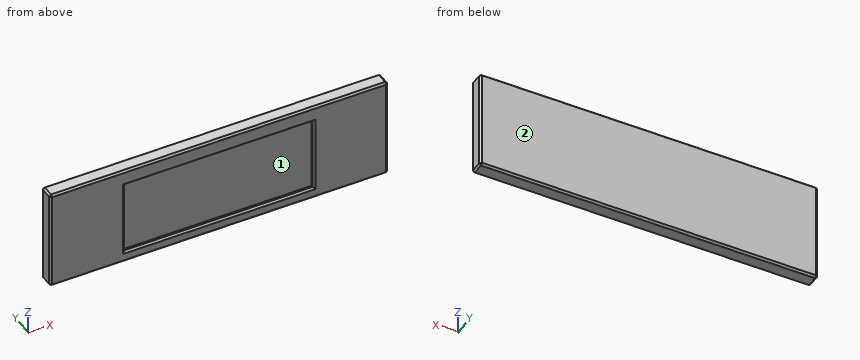
from build123d import *

# Parameters (mm, degrees)
F0_W     = 900
F0_H     = 270
F0_W_2   = 502
F0_H_2   = 197
F1_DEPTH = 40
F2_DEPTH = 30
F3_SIZE  = 5


with BuildPart() as f1:
    # F0 (on Front) → F1 (new body)
    with BuildSketch(Plane.XZ):
        with Locations((-14.222194, -51.038729)):
            Rectangle(F0_W, F0_H)
        with Locations((-13.586061, -57.538729)):
            Rectangle(F0_W_2, F0_H_2, mode=Mode.SUBTRACT)
    extrude(amount=F1_DEPTH)

    # F0 (on Front) → F2 (join)
    with BuildSketch(Plane.XZ):
        with Locations((-13.586061, -57.538729)):
            Rectangle(F0_W_2, F0_H_2)
    extrude(amount=F2_DEPTH)

    # F3
    f3_edges = [f1.edges().sort_by_distance(p)[0] for p in [
        (435.777806, -40, -51.038729),
        (-14.222194, -40, 83.961271),
        (-464.222194, -40, -51.038729),
        (-14.222194, -40, -186.038729),
        (-264.586061, -40, -57.538729),
        (-13.586061, -40, 40.961271),
        (237.413939, -40, -57.538729),
        (-13.586061, -40, -156.038729),
        (-464.222194, -20, 83.961271),
        (-464.222194, -20, -186.038729),
        (-464.222194, 0, -51.038729),
        (435.777806, -20, -186.038729),
        (435.777806, -20, 83.961271),
        (435.777806, 0, -51.038729),
        (-14.222194, 0, -186.038729),
        (-14.222194, 0, 83.961271),
    ]]
    chamfer(f3_edges, length=F3_SIZE)


solid = f1.part
Verification items for the finished model (mm, model axes). Face numbers are marked on the shaded views. A direction names the side the tool comes from. Coordinates: 2 decimals unless noted, no trailing zeros. Order: outer loops, then holes, each group sorted by start corner. A loop starts at its lowest first (then second) coordinate and runs counter-clockwise, first axis right, second up. Notation, with made-up numbers: M -37.5,-11 L 21.5,-11 A13 ccw 21.5,-1 Z; hole C -35.75,72 d2. An arc over 180 degrees is marked long. One line per item, written item: value. Start each with the question number.
Item 1: Sectioned sample at A-A (z = -15). Enter the section's corners in (x, y).
Item 2: Gauge pin test, flat end, axial feed: pin 1 (1 mm diameter, centred on x = -98, z = 9, fed in from -Y). Record the tip position at first contact, or that the pin passes through.
Item 3: Access from +Z, -Z, +X, -X, +Y, -Y to the whole of each face (thin tool, end or side, straight path). Record for the marked faces 1 and 2.
Item 4: Scan lines: probe 1 along Z at (x, y) = (-131, -34); probe 2 along X at (y, z) = (-32, -36); probe 3 along Z at (x, y) = (220, -36.5). Record each from-to range of solid material in increasing order.
Conclusion:
1. outline: M -464.22,-35 L -459.22,-40 L -269.59,-40 L -264.59,-35 L -264.59,-30 L 237.41,-30 L 237.41,-35 L 242.41,-40 L 430.78,-40 L 435.78,-35 L 435.78,-5 L 430.78,0 L -459.22,0 L -464.22,-5 Z
2. pin 1: stops at y = -30
3. face 1: -Y
3. face 2: +Z, -Z, +X, -X, +Y
4. probe 1: z = -186.04 to -156.04, 40.96 to 83.96
4. probe 2: x = -464.22 to -264.59, 237.41 to 435.78
4. probe 3: z = -184.54 to -157.54, 42.46 to 82.46
